Model file for the job. Use its own axes, mm. Face numbers are marked on the shaded views. A direction names the side the tool comes from. Give positions to 0.01 mm unless a question says otherwise; leave off trailing zeros. Loops run counter-clockwise (first coordinate to the right, second up) from the corner with the lowest first, then second, coordinate; pieces in that order, holes last. Notation, with made-up numbers: (88.5, 17.25) - (107.5, 17.25) arc R13 ccw to (107.5, 37.25) - close; hole circle Ø8 at (-32.75, 42). An arc over 180 degrees is marked (long way). Use a Markdown table: item, result.
from build123d import *

# Parameters (mm, degrees)
BOSS_EXTRUDE1_DEPTH = 3.3
BOSS_EXTRUDE2_DEPTH = 1
SKETCH4_R           = 2.75
CUT_EXTRUDE1_DEPTH  = 5.3
CUT_EXTRUDE2_DEPTH  = 7
FILLET1_R           = 0.4


with BuildPart() as part:
    # Sketch1 → Boss-Extrude1 (new body)
    with BuildSketch(Plane(origin=(0, 0, 0), x_dir=(1, 0, 0), z_dir=(0, 1, 0))):
        with BuildLine():
            Line((-5, -3), (4, -3))
            ThreePointArc((4, -3), (4.74341641, -1.581139071), (5, -5.07e-07))
            Line((5, -5.07e-07), (5, 3))
            Line((5, 3), (-4, 3))
            ThreePointArc((-4, 3), (-4.74341641, 1.581139071), (-5, 5.07e-07))
            Line((-5, 5.07e-07), (-5, -3))
        make_face()
    extrude(amount=BOSS_EXTRUDE1_DEPTH)

    # Sketch3 → Boss-Extrude2 (add)
    with BuildSketch(Plane(origin=(0, 3.3, 0), x_dir=(1, 0, 0), z_dir=(0, 1, 0))):
        with BuildLine():
            Line((-3, -3), (1.443496021, -3))
            ThreePointArc((1.443496021, -3), (2.424601601, -1.998754321), (3, -0.720482929))
            Line((3, -0.720482929), (3, 3))
            Line((3, 3), (-1.352396976, 3))
            ThreePointArc((-1.352396976, 3), (-2.373272189, 2.039336237), (-3, 0.785433003))
            Line((-3, 0.785433003), (-3, -3))
        make_face()
    extrude(amount=BOSS_EXTRUDE2_DEPTH)

    # Sketch4 → Cut-Extrude1 (cut, through all)
    with BuildSketch(Plane(origin=(0, 4.3, 0), x_dir=(1, 0, 0), z_dir=(0, 1, 0))):
        Circle(SKETCH4_R)
    extrude(amount=-CUT_EXTRUDE1_DEPTH, mode=Mode.SUBTRACT)

    # Sketch5 → Cut-Extrude2 (cut, through all)
    with BuildSketch(Plane.XY.offset(3)):
        Polygon((4, 0), (5, 0), (5, 2.185994227), (3.604159787, 0), align=None)
        Polygon((-5, 0), (-3.604159787, 0), (-5, 2.185994227), align=None)
    extrude(amount=-CUT_EXTRUDE2_DEPTH, mode=Mode.SUBTRACT)

    # Fillet1
    fillet1_edges = [part.edges().sort_by_distance(p)[0] for p in [
        (-5, 2.742997113, 3),
        (5, 2.742997113, -3),
        (-4.74341641, 3.3, -1.581139071),
        (-5, 3.3, 1.499999746),
        (3, 3.8, -3),
        (4.74341641, 3.3, 1.581139071),
        (-3, 3.8, 3),
        (5, 3.3, -1.499999746),
    ]]
    fillet(fillet1_edges, radius=FILLET1_R)


solid = part.part
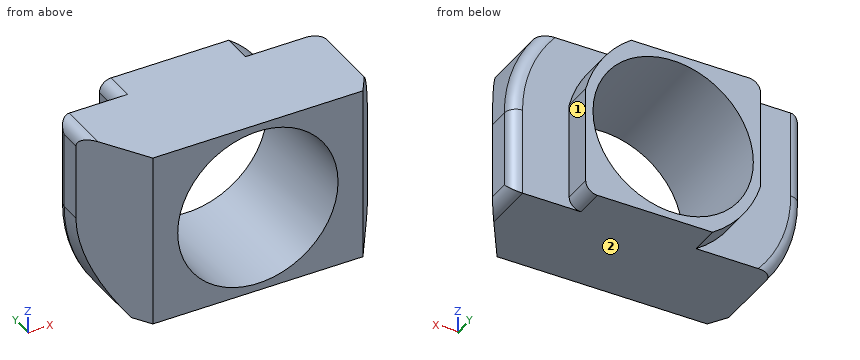
(1) Slice it at C-C, the plane x = -2.5. Write the cut outline in (y, z), plus the area to 3 significant figures.
Computed:
| item | result |
|---|---|
| outline | (0, -3) - (3.3, -3) - (3.3, -1.86) - (4.3, -1.86) - (4.3, -1.15) - (0, -1.15) - close; (0, 1.15) - (4.3, 1.15) - (4.3, 3) - (0, 3) - close |
| area | 14.8 mm² |
(2) Drill centre lines: probe 1 along Z at (x, y) = (0, 2.7); probe 2 along X at (y, z) = (2.4, 0); probe 3 along Y at (x, z) = (-2.5, -2.5). Where is each one in solid material? Low to high. Write a range as [from, to].
Computed:
| item | result |
|---|---|
| probe 1 | [-3, -2.75], [2.75, 3] |
| probe 2 | [-5, -2.75], [2.75, 5] |
| probe 3 | [0, 3.3] |
(3) Slice it at A-A, the plane x = 0. Write the cut outline in (y, z), plus the area to 3 significant figures.
Computed:
| item | result |
|---|---|
| outline | (0, -3) - (4.3, -3) - (4.3, -2.75) - (0, -2.75) - close; (0, 2.75) - (4.3, 2.75) - (4.3, 3) - (0, 3) - close |
| area | 2.15 mm² |
(4) Slice it at B-B, the plane y = 3.75. Write the cut outline in (x, z).
Computed:
| item | result |
|---|---|
| outline | (-3, -0.79) arc R4 ccw to (-1.35, -3) - (2.6, -3) arc R0.4 ccw to (3, -2.6) - (3, 0.72) arc R4 ccw to (1.44, 3) - (-2.6, 3) arc R0.4 ccw to (-3, 2.6) - close; hole circle Ø5.5 at (0, 0) |
(5) Slice it at D-D, the plane y = 3.1. Write the cut outline in (x, z).
Computed:
| item | result |
|---|---|
| outline | (-4.95, 0) arc R4.95 ccw to (-3.93, -3) - (4.6, -3) arc R0.4 ccw to (4.95, -2.8) - (4.95, 0) arc R4.95 ccw to (3.93, 3) - (-4.6, 3) arc R0.4 ccw to (-4.95, 2.8) - close; hole circle Ø5.5 at (0, 0) |
(6) Pin check, flat tips, straight feed: P1, Ø0.8, axis at y = 4, z = 0.5, coming from the -X side; P2, Ø1.5, axis at x = -3.5, z = -0.5, coming from the -Y side; P3, Ø0.5, axis at y = 4, z = -1.5, coming from the +X side; P4, Ø1, axis at x = -3.5, z = -1, coming from the +Y side. Stop position of each tip, or through.
Computed:
| item | result |
|---|---|
| P1 | x = -3 |
| P2 | y = 0 |
| P3 | x = 3 |
| P4 | y = 3.3 |
(7) 3-axis set-ups, long thin cutter, end or side, ignore diameter. For the marked faces 1 and 2: which of +Z, -Z, +X, -X, +Y, -Y reach the whole face in a straight line?
Computed:
| item | result |
|---|---|
| face 1 | +Z, -Z, +X, +Y |
| face 2 | -Z, +X, -X, +Y, -Y |
